Verification items for this drawing (mm, ordinates from the low corner). Round coordinates to 2 decimals unless told otherwise and drop trailing zeros. Loops run counter-clockwise (first coordinate to the right, second up) from the corner with the lowest first, then second, coordinate; pieces in that order, holes last. Notation, with made-up numbers: M 16,54 L 55,54 A13 ccw 55,71 Z; hole C -12,54 d9. An arc over 180 degrees is marked long. Use one line per item in the form item = value. Start each with the question number.
1. Draft check along Z on the marked faces 1, 2 and 3. Enter one of: pulls with the +Z half, pulls with the -Z half, needs draft (parallel to the pull), parting line crosses it, or undercut.
2. Cross-section at C-C (x = 65). State how many separate pieces and enclosed holes the cut face has, then the cut area to 3 significant figures.
3. Cross-section at B-B (x = 82.55). Record the boundary of the cut face in (y, z) (1 decimal), then the cut area to 3 significant figures.
4. Go/stop test with flat-tipped pins: pin 1 (5 mm diameter, centred on x = 23.5, z = 41.5, fed in from +Y); pin 2 (1.5 mm diameter, centred on y = 6, z = 67, fed in from -X); pin 3 (8 mm diameter, centred on y = 18, z = 59.5, fed in from -X); pin 4 (2 mm diameter, centred on y = 3.5, z = 32, fed in from -X). Record where each tip stops, or that it passes through.
5. Cross-section at A-A (z = 50.8). Record the boundary of the cut face in (x, y) (1 decimal).
6. Cross-section at D-D (z = 27). Record the boundary of the cut face in (x, y), then the cut area to 3 significant figures.
7. Material ranges on line 1 (Z direction, x = 54, y = 13.75); line 2 (X direction, y = 3.75, z = 74.5) (1 decimal); line 3 (X direction, y = 1.75, z = 30.5), recorded low to high.
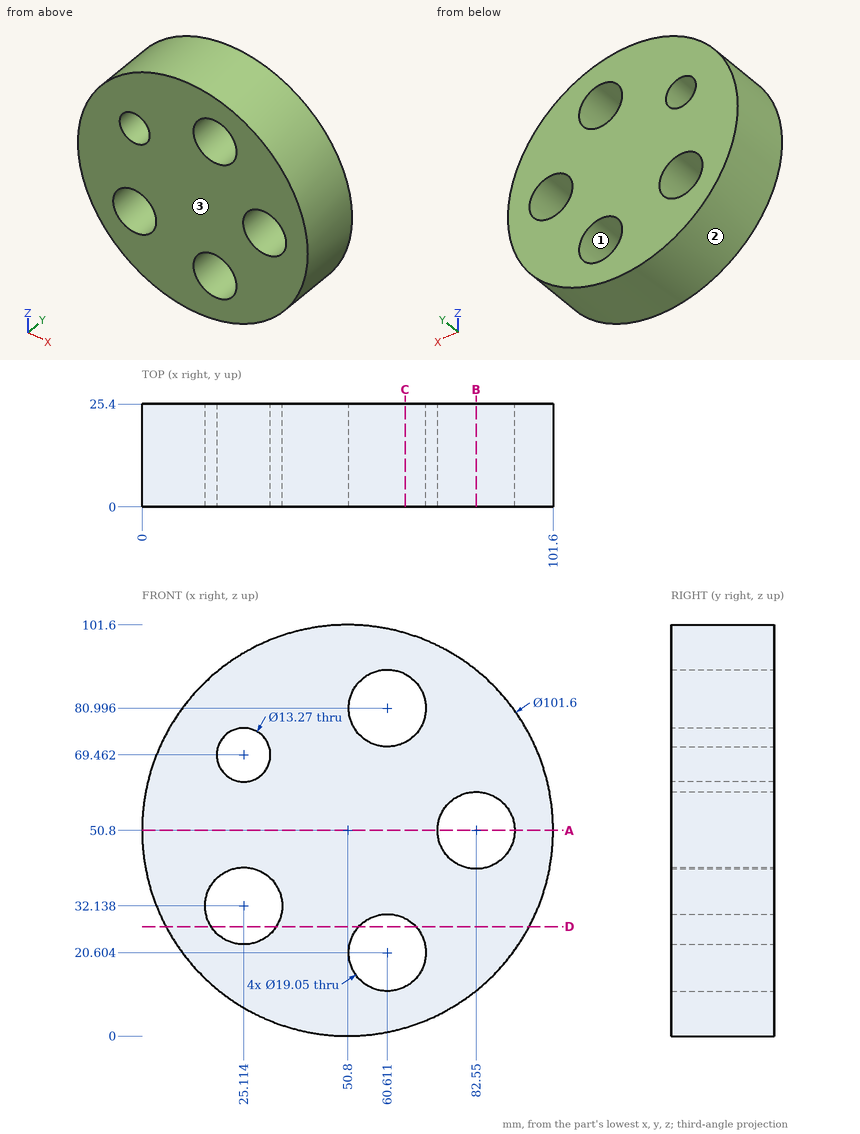
Reported:
q1.face_1 = undercut
q1.face_2 = parting line crosses it
q1.face_3 = needs draft
q2.separate_pieces = 3
q2.enclosed_holes = 0
q2.area = 1,620 mm²
q3.outline = M 0,11.1 L 25.4,11.1 L 25.4,41.3 L 0,41.3 Z; M 0,60.3 L 25.4,60.3 L 25.4,90.5 L 0,90.5 Z
q3.area = 1,530 mm²
q4.pin_1 = 25.4
q4.pin_2 = 2.41
q4.pin_3 = 0.22
q4.pin_4 = 3.22
q5.outline = M 0,0 L 73,0 L 73,25.4 L 0,25.4 Z; M 92.1,0 L 101.6,0 L 101.6,25.4 L 92.1,25.4 Z
q6.outline = M 5.92,0 L 17.09,0 L 17.09,25.4 L 5.92,25.4 Z; M 33.13,0 L 53.55,0 L 53.55,25.4 L 33.13,25.4 Z; M 67.67,0 L 95.68,0 L 95.68,25.4 L 67.67,25.4 Z
q6.area = 1,510 mm²
q7.line_1 = 0.1 to 13.75, 27.46 to 74.14, 87.85 to 101.5
q7.line_2 = 5.9 to 20.8, 29.4 to 53.6, 67.6 to 95.7
q7.line_3 = 4.23 to 15.73, 34.5 to 97.37
